Could you check a few things on this model? Use its own coordinates, in mm. A direction names the side the tool comes from. Coordinates: 2 decimals unless noted, no trailing zeros. Order: outer loops, then holes, each group sorted by start corner. A loop starts at its lowest first (then second) coordinate and runs counter-clockwise, first axis right, second up.
```python
from build123d import *

# Parameters (mm, degrees)
BASEHEAD_DEPTH = 6.8072


with BuildPart() as part:
    # Sketch1 → BaseHead (new body)
    with BuildSketch(Plane(origin=(0, 0, 0), x_dir=(0, 0, -1), z_dir=(1, 0, 0))):
        Polygon((7.1374, 4.120779811), (7.1374, -4.120779811), (0, -8.241559623), (-7.1374, -4.120779811), (-7.1374, 4.120779811), (0, 8.241559623), align=None)
    extrude(amount=BASEHEAD_DEPTH)

    # BodySke → BaseBody (revolve)
    with BuildSketch(Plane.XY):
        Polygon((0, 0), (44.9072, 0), (44.9072, 4.13258), (44.27728, 4.7625), (0, 4.7625), align=None)
    revolve(axis=Axis((0, 0, 0), (1, 0, 0)))

    # Sketch3 → HeadChamfer (revolve, cut)
    with BuildSketch(Plane.XY):
        Polygon((0, 7.1374), (4.303661065, 14.591559623), (4.303661065, 20.941559623), (-12.7, 20.941559623), (-12.7, 7.1374), align=None)
    revolve(axis=Axis((0, 0, 0), (1, 0, 0)), mode=Mode.SUBTRACT)


solid = part.part
```
Item 1: For pin 1 Ø1.5 at (x, z) = (17, 4) entering from -Y; pin 2 Ø4 at (x, y) = (25, -3.5) entering from -Z; pin 3 Ø5 at (x, y) = (24.5, 0.5) entering from -Z, each with a flat end and sliding along its axis, tell me the tip position at first contact or that it passes through.
Item 2: Suppose I cut it at A-A (x = 38.5). List the corners of the cut face in (y, z) for me (1 decimal).
Item 3: Which directions (+Z, -Z, +X, -X, +Y, -Y) give clear straight access to the entire face, cutting with the end or side of a thin tool? Please do faces 1 (the face through (3.36, -6.15, -3.62)), 2 (the face through (25.28, -3.78, -2.9)).
Item 4: I need wall thicknesses on line 1 (X direction, y = -2.5, z = -4.75); line 2 (Y direction, x = 40.5, z = 0); line 3 (Y direction, x = 25, z = 1.25). Which ranges of each line are inside material? Lowest first, please.
Geometry results:
1. pin 1: stops at y = -3.48
1. pin 2: stops at z = -4.52
1. pin 3: stops at z = -4.76
2. outline: circle Ø9.5 at (0, 0)
3. face 1: -Z, +X, -X, -Y
3. face 2: +X
4. line 1: x = 0 to 6.81
4. line 2: y = -4.76 to 4.76
4. line 3: y = -4.6 to 4.6
